For this review, take the finished solid that the model builds, in its own axes (mm). A direction names the side the tool comes from. Coordinates: 2 decimals unless noted, no trailing zeros. Write each loop counter-clockwise with the first axis right and the second up, starting at its lowest first coordinate (ties: lowest second). Pieces come first, ordered by that corner, then holes.
```python
from build123d import *

# Parameters (mm, degrees)
F0_W     = 1016
F0_H     = 1905
F1_DEPTH = 1016
F2_W     = 1016
F2_H     = 713.0777835846
F3_DEPTH = 635
F4_R     = 106.5109159408
F5_DEPTH = 193.04
F6_R     = 64.5918203827
F7_DEPTH = 127


# Not quite as in the source:
# - the program builds the solid bodies; features that only make, move or delete a surface that nothing else refers to are left out


with BuildPart() as f1:
    # F0 (on Front) → F1 (new body)
    with BuildSketch(Plane.XZ):
        with Locations((-508, 952.5)):
            Rectangle(F0_W, F0_H)
    extrude(amount=F1_DEPTH)

    # F2 (on face) → F3 (cut)
    with BuildSketch(Plane.XZ.offset(1016)):
        with Locations((-508, 1121.7548847198)):
            Rectangle(F2_W, F2_H)
    extrude(amount=-F3_DEPTH, mode=Mode.SUBTRACT)

    # F4 (on face) → F5 (join)
    with BuildSketch(Plane(origin=(0, 0, 1478.2937765121), x_dir=(1, 0, 0), z_dir=(0, 0, -1))):
        with Locations((-495.6358075142, 729.4123768806)):
            Circle(F4_R)
    extrude(amount=F5_DEPTH)

    # F6 (on face) → F7 (join)
    with BuildSketch(Plane(origin=(0, 0, 1285.2537765121), x_dir=(1, 0, 0), z_dir=(0, 0, -1))):
        with Locations((-495.6358075142, 729.4123768806)):
            Circle(F6_R)
    extrude(amount=F7_DEPTH)


solid = f1.part
```
Q1. Tool access review of faces 4 (the flat face through (-515, -501, 0)), 5 (the flat face through (-497, -730, 1158.254)), 6 (the flat face through (-449.8, -683.6, 1285.254)): name each direction out of +Z, -Z, +X, -X, +Y, -Y from which nothing blocks a thin tool from reaching the whole face with its end or side.
Ans:
face 4: -Z, +X, -X, +Y, -Y
face 5: +X, -X, -Y
face 6: none
Q2. For probe 1 along Z at (x, y) = (-827, -387); probe 2 along Y at (x, z) = (-652.5, 932.5), list the stretches that pass through material, from the lowest coordinate up.
Ans:
probe 1: z = 0 to 765.22, 1478.29 to 1905
probe 2: y = -381 to 0
Q3. Add section C-C (z = 1444.5). State the section outline as (x, y) points, then the cut area to 3 significant figures.
Ans:
outline: (-1016, -381) - (0, -381) - (0, 0) - (-1016, 0) - close; circle Ø213.02 at (-495.64, -729.41)
area: 423,000 mm2
Q4. Add section D-D (y = -689). State the section outline as (x, z) points, then the cut area to 3 significant figures.
Ans:
outline: (-1016, 0) - (0, 0) - (0, 765.22) - (-1016, 765.22) - close; (-1016, 1478.29) - (-594.18, 1478.29) - (-594.18, 1285.25) - (-546.02, 1285.25) - (-546.02, 1158.25) - (-445.25, 1158.25) - (-445.25, 1285.25) - (-397.09, 1285.25) - (-397.09, 1478.29) - (0, 1478.29) - (0, 1905) - (-1016, 1905) - close
area: 1,260,000 mm2
Q5. Add section A-A (y = -482). State the section outline as (x, z) points.
Ans:
outline: (-1016, 0) - (0, 0) - (0, 765.22) - (-1016, 765.22) - close; (-1016, 1478.29) - (0, 1478.29) - (0, 1905) - (-1016, 1905) - close
Q6. Add section B-B (x = -848). State the section outline as (y, z) points, then the cut area to 3 significant figures.
Ans:
outline: (-1016, 0) - (0, 0) - (0, 1905) - (-1016, 1905) - (-1016, 1478.29) - (-381, 1478.29) - (-381, 765.22) - (-1016, 765.22) - close
area: 1,480,000 mm2
Q7. Draft analysis for pull direction Z (two halves, no side actions). For faces 1 (the flat face through (-515, -501, 1905)), 2 (the flat face through (-515, 0, 966)), 3 (the cylindrical face through (-580.16, -664.6, 1383.13)), state which applies: +Z half, -Z half, draft (parallel to the pull), parting line (faces both ways), or undercut.
Ans:
face 1: +Z half
face 2: draft
face 3: undercut
Q8. Clearance check with flat-ended pins moving along their axes: pin 1 Ø5 at (y, z) = (-691, 549) entering from +X; pin 2 Ø6 at (x, z) = (-276.5, 1199.5) entering from -Y. State where each tip first meets the part, or that it passes through.
Ans:
pin 1: stops at x = 0
pin 2: stops at y = -381
